Source: CAD feature listing. Evaluate the final solid. Frame: model axes, mm. A direction names the side the tool comes from. Give positions to 0.01 mm unless a question says otherwise; leave off trailing zeros. Order: outer loops, then holes, each group sorted by start corner. A loop starts at its lowest first (then second) coordinate and runs counter-clockwise, first axis right, second up. Notation, with made-up numbers: M 65.5,25.5 L 93.5,25.5 A21 ccw 93.5,50.5 Z; hole C 79,79.5 d3. An arc over 180 degrees is marked long. Answer as a JSON object with one key per item and string values. Group by question number.
1. Section query A-A (x = -6). Output: boundary loops of the cut face in (y, z), plus the area to 3 significant figures.
2. Section query C-C (z = 8.5). Output: boundary loops of the cut face in (x, y).
3. Pin query (flat end, axial travel): P1, Ø5, axis at x = -4, y = 14.5, coming from the -Z side. Return the tip coordinate at first contact, or that it passes through.
4. Pull-direction query (Y, two-part tool) for faces 1 (the flat face through (-7, 15.189, 8)), 2 (the flat face through (-7, 16, 10)), 3 (the flat face through (-7, 18.589, 5)); classes: +Y half, -Y half, draft (parallel to the pull), parting line (faces both ways), or undercut.
5. Section query D-D (y = 14.5). Output: boundary loops of the cut face in (x, z).
6. Set-up query: faces 4 (the flat face through (-7, 10.589, 3)), 5 (the flat face through (-7, 11.989, 8)), 6 (the flat face through (-26.818, 14, 5)). Return all of +Z, -Z, +X, -X, +Y, -Y with unobstructed straight access to the full face (end or side cutting, diameter ignored); none if empty.
7. Material intervals for L1, parallel to Y at x = -6.5, z = 1; L2, parallel to Y at x = -10, z = 9; L3, parallel to X at y = 12.5, z = 1.25, sorted ascending. Write a range as [from, to].
8. Section query B-B (y = 13). Output: boundary loops of the cut face in (x, z).
from build123d import *

# Parameters (mm, degrees)
SKETCH_1_W          = 40
SKETCH_1_H          = 10
SKETCH_1_R          = 1.6
EXTRUDE_1_DEPTH     = 10
SKETCH_2_W          = 20
SKETCH_2_H          = 6
CUT_EXTRUDE_1_DEPTH = 6


with BuildPart() as part:
    # 草图1 → 凸台-拉伸1 (new body)
    with BuildSketch(Plane.XY):
        with Locations((-6.818181818, 13.588516746)):
            Rectangle(SKETCH_1_W, SKETCH_1_H)
        with Locations((-21.818181818, 13.588516746)):
            Circle(SKETCH_1_R, mode=Mode.SUBTRACT)
        with Locations((8.181818182, 13.588516746)):
            Circle(SKETCH_1_R, mode=Mode.SUBTRACT)
        with BuildLine():
            Line((-14.318181818, 15.188516746), (0.681818182, 15.188516746))
            ThreePointArc((0.681818182, 15.188516746), (2.281818182, 13.588516746), (0.681818182, 11.988516746))
            Line((0.681818182, 11.988516746), (-14.318181818, 11.988516746))
            ThreePointArc((-14.318181818, 11.988516746), (-15.918181818, 13.588516746), (-14.318181818, 15.188516746))
        make_face(mode=Mode.SUBTRACT)
    extrude(amount=EXTRUDE_1_DEPTH)

    # 草图2 → 切除-拉伸1 (cut)
    with BuildSketch(Plane(origin=(0, 0, 0), x_dir=(-1, 0, 0), z_dir=(0, 0, -1))):
        with Locations((6.818181818, 13.588516746)):
            Rectangle(SKETCH_2_W, SKETCH_2_H)
    extrude(amount=-CUT_EXTRUDE_1_DEPTH, mode=Mode.SUBTRACT)


solid = part.part
Answer sheet:
{
 "1": {"outline": "M 8.59,0 L 10.59,0 L 10.59,6 L 11.99,6 L 11.99,10 L 8.59,10 Z; M 15.19,6 L 16.59,6 L 16.59,0 L 18.59,0 L 18.59,10 L 15.19,10 Z", "area": "51.2 mm^2"},
 "2": {"outline": "M -26.82,8.59 L 13.18,8.59 L 13.18,18.59 L -26.82,18.59 Z; hole C -21.82,13.59 d3.2; hole M -14.32,11.99 L 0.68,11.99 A1.6 ccw 0.68,15.19 L -14.32,15.19 A1.6 ccw Z; hole C 8.18,13.59 d3.2"},
 "3": {"P1": "z = 0"},
 "4": {"face 1": "undercut", "face 2": "draft", "face 3": "+Y half"},
 "5": {"outline": "M -26.82,0 L -23.13,0 L -23.13,10 L -26.82,10 Z; M -20.5,0 L -16.82,0 L -16.82,6 L -15.63,6 L -15.63,10 L -20.5,10 Z; M 2,6 L 3.18,6 L 3.18,0 L 6.87,0 L 6.87,10 L 2,10 Z; M 9.5,0 L 13.18,0 L 13.18,10 L 9.5,10 Z"},
 "6": {"face 4": "-Z", "face 5": "+Z, -Z", "face 6": "+Z, -Z, -X, +Y, -Y"},
 "7": {"L1": "[8.59, 10.59], [16.59, 18.59]", "L2": "[8.59, 11.99], [15.19, 18.59]", "L3": "[-26.82, -22.99], [-20.65, -16.82], [3.18, 7.01], [9.35, 13.18]"},
 "8": {"outline": "M -26.82,0 L -23.31,0 L -23.31,10 L -26.82,10 Z; M -20.33,0 L -16.82,0 L -16.82,6 L -15.81,6 L -15.81,10 L -20.33,10 Z; M 2.17,6 L 3.18,6 L 3.18,0 L 6.69,0 L 6.69,10 L 2.17,10 Z; M 9.67,0 L 13.18,0 L 13.18,10 L 9.67,10 Z"}
}
